from build123d import *
from build123d.topology import SkipClean

# Parameters (mm, degrees)
SKETCH_1_R          = 15
SKETCH_1_R_2        = 7
EXTRUDE_1_DEPTH     = 2.6
SKETCH_2_R          = 15
SKETCH_2_R_2        = 4
EXTRUDE_2_DEPTH     = 10.8
SKETCH_3_R          = 15
SKETCH_3_R_2        = 7
EXTRUDE_3_DEPTH     = 2.6
EXTRUDE_START       = 0.8
SKETCH_4_R          = 15
SKETCH_4_R_2        = 8
EXTRUDE_4_DEPTH     = 0.8
SKETCH_5_R          = 15
SKETCH_5_R_2        = 8
EXTRUDE_5_DEPTH     = 0.8
SKETCH_6_R          = 4.1
CUT_EXTRUDE_1_DEPTH = 30


with BuildPart() as part:
    # Sketch 1 → Extrude 1 (new body)
    with BuildSketch(Plane.XY):
        Circle(SKETCH_1_R)
        Circle(SKETCH_1_R_2, mode=Mode.SUBTRACT)
    extrude(amount=EXTRUDE_1_DEPTH)

    # Sketch 2 → Extrude 2 (add)
    with BuildSketch(Plane.XY.offset(2.6)):
        Circle(SKETCH_2_R)
        with Locations(Location((0, 0, 0), (0, 0, 180))):
            Circle(SKETCH_2_R_2, mode=Mode.SUBTRACT)
    extrude(amount=EXTRUDE_2_DEPTH)

    # Sketch 3 → Extrude 3 (add)
    with BuildSketch(Plane.XY.offset(13.4)):
        Circle(SKETCH_3_R)
        Circle(SKETCH_3_R_2, mode=Mode.SUBTRACT)
    extrude(amount=EXTRUDE_3_DEPTH)

    # Sketch 4 → Extrude 4 (add)
    with SkipClean():  # the faces are left unmerged after this step: merging them gives an invalid solid
        with BuildSketch(Plane(origin=(0, 0, 0), x_dir=(-1, 0, 0), z_dir=(0, 0, -1)).offset(EXTRUDE_START)):
            Circle(SKETCH_4_R)
            Circle(SKETCH_4_R_2, mode=Mode.SUBTRACT)
        extrude(amount=-EXTRUDE_4_DEPTH)

    # Sketch 5 → Extrude 5 (add)
    with BuildSketch(Plane.XY.offset(16)):
        with Locations(Location((0, 0, 0), (0, 0, 180))):
            Circle(SKETCH_5_R)
        with Locations(Location((0, 0, 0), (0, 0, 180))):
            Circle(SKETCH_5_R_2, mode=Mode.SUBTRACT)
    extrude(amount=EXTRUDE_5_DEPTH)

    # Sketch 6 → Cut-Extrude 1 (cut)
    with BuildSketch(Plane(origin=(0, 0, 2.6), x_dir=(-1, 0, 0), z_dir=(0, 0, -1))):
        Circle(SKETCH_6_R)
    extrude(amount=-CUT_EXTRUDE_1_DEPTH, mode=Mode.SUBTRACT)


solid = part.part
Design review of the part built by this model. Coordinates are the model's own, in mm. A direction names the side the tool comes from. Coordinates: 2 decimals unless noted, no trailing zeros. Order: outer loops, then holes, each group sorted by start corner. A loop starts at its lowest first (then second) coordinate and runs counter-clockwise, first axis right, second up. Notation, with made-up numbers: (19, 66.5) - (42, 66.5) arc R28 ccw to (42, 85.5) - close; hole circle Ø8 at (-33.75, -22). An arc over 180 degrees is marked (long way). Put each result on its own line as item: value.
1) Tool access review of faces 1 (the face through (4, -6, 0)), 2 (the face through (3.01, -3.01, 13.4)), 3 (the face through (-6, -6, -0.8)): name each direction out of +Z, -Z, +X, -X, +Y, -Y from which nothing blocks a thin tool from reaching the whole face with its end or side.
Response values:
face 1: -Z
face 2: +Z
face 3: -Z, +X, -X, +Y, -Y
2) Wall thickness on L1, parallel to Y at x = 0, z = -0.6; L2, parallel to Y at x = 0, z = 1.3; L3, parallel to X at y = -1, z = 7.5: over which ranges is each line inside the solid? List them lowest first. Write a range as from..to.
Response values:
L1: y = -15..-8, 8..15
L2: y = -15..-7, 7..15
L3: x = -14.97..-3.98, 3.98..14.97
3) Insertion check: P1, Ø4, axis at x = -3, y = -2, coming from the +Z side; P2, Ø13, axis at x = 0.5, y = -0.5, coming from the +Z side; P3, Ø10, axis at y = 8, z = 8.5, coming from the -X side. Each pin has a flat end and moves straight along its axis. Give the tip position at first contact, or say it passes through.
Response values:
P1: stops at z = 13.4
P2: stops at z = 16
P3: stops at x = -14.7
4) The part is to be moulded in two halves that separate along Y. For faces 4 (the face through (-6, 6, 16.8)), 5 (the face through (3.01, -3.01, 2.6)), 6 (the face through (4, -6, 16)), say which applies: released by +Y, released by -Y, zero draft, split by the parting line, or undercut.
Response values:
face 4: zero draft
face 5: undercut
face 6: undercut
5) Take a section at C-C, the plane z = 6.75. Give the boundary of the cut face in (x, y).
Response values:
outline: circle Ø30 at (0, 0); hole circle Ø8.2 at (0, 0)
6) Take a section at A-A, the plane x = 0. Give the boundary of the cut face in (y, z), and give its area (3 significant figures).
Response values:
outline: (-15, -0.8) - (-8, -0.8) - (-8, 0) - (-7, 0) - (-7, 2.6) - (-4.1, 2.6) - (-4.1, 13.4) - (-7, 13.4) - (-7, 16) - (-8, 16) - (-8, 16.8) - (-15, 16.8) - close; (4.1, 2.6) - (7, 2.6) - (7, 0) - (8, 0) - (8, -0.8) - (15, -0.8) - (15, 16.8) - (8, 16.8) - (8, 16) - (7, 16) - (7, 13.4) - (4.1, 13.4) - close
area: 341 mm²
7) Take a section at D-D, the plane x = -4.75. Give the boundary of the cut face in (y, z).
Response values:
outline: (-14.23, -0.8) - (-6.44, -0.8) - (-6.44, 0) - (-5.14, 0) - (-5.14, 2.6) - (5.14, 2.6) - (5.14, 0) - (6.44, 0) - (6.44, -0.8) - (14.23, -0.8) - (14.23, 16.8) - (6.44, 16.8) - (6.44, 16) - (5.14, 16) - (5.14, 13.4) - (-5.14, 13.4) - (-5.14, 16) - (-6.44, 16) - (-6.44, 16.8) - (-14.23, 16.8) - close
